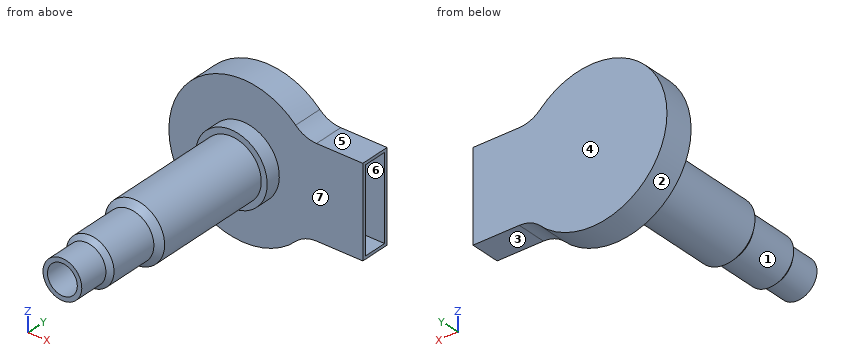
```python
from build123d import *

# Parameters (mm, degrees)
BOSS_EXTRUDE1_DEPTH = 10
SHELL1_T            = -1


with BuildPart() as part:
    # Sketch1 → Revolve1 (revolve)
    with BuildSketch(Plane(origin=(0, 0, 0), x_dir=(0, 0, -1), z_dir=(1, 0, 0))):
        Polygon((5, 0), (6.5, 0), (6.5, 10), (8, 11.5), (8, 28), (10, 30), (10, 70), (12, 70), (12, 75), (0, 75), (0, 35), (5, 35), align=None)
    revolve(axis=Axis((0, 0, 0), (0, 1, 0)))


with BuildPart() as body_2:
    # Sketch2 → Boss-Extrude1 (new body)
    with BuildSketch(Plane(origin=(0, 75, 0), x_dir=(1, 0, 0), z_dir=(0, 1, 0))):
        with BuildLine():
            Line((24.494897428, 15), (40, 15))
            Line((40, 15), (40, -15))
            Line((40, -15), (24.494897428, -15))
            ThreePointArc((24.494897428, -15), (20.715252698, -15.741799002), (17.496355306, -17.857142857))
            ThreePointArc((17.496355306, -17.857142857), (-25, 0), (17.496355306, 17.857142857))
            ThreePointArc((17.496355306, 17.857142857), (20.715252698, 15.741799002), (24.494897428, 15))
        make_face()
    extrude(amount=BOSS_EXTRUDE1_DEPTH)

    # Shell1
    shell1_openings = [body_2.faces().sort_by_distance(p)[0] for p in [
        (40, 80, 0),
    ]]
    offset(amount=SHELL1_T, openings=shell1_openings, kind=Kind.INTERSECTION)

    # Combine1: union part
    add(part.part)


solid = body_2.part
```
Source: CAD feature listing. Evaluate the final solid. Frame: model axes, mm. Face numbers are marked on the shaded views. A direction names the side the tool comes from. Round coordinates to 2 decimals unless told otherwise and drop trailing zeros. Loops run counter-clockwise (first coordinate to the right, second up) from the corner with the lowest first, then second, coordinate; pieces in that order, holes last.
(1) Section query C-C (z = -19.5). Output: boundary loops of the cut face in (x, y).
From the geometry:
outline: (-15.64, 75) - (15.64, 75) - (15.64, 85) - (-15.64, 85) - close; hole (-13.99, 76) - (13.99, 76) - (13.99, 84) - (-13.99, 84) - close
(2) Section query B-B (z = 0). Output: boundary loops of the cut face in (x, y), and give its area (3 significant figures).
From the geometry:
outline: (-25, 75) - (-12, 75) - (-12, 70) - (-10, 70) - (-10, 30) - (-8, 28) - (-8, 11.5) - (-6.5, 10) - (-6.5, 0) - (-5, 0) - (-5, 35) - (5, 35) - (5, 0) - (6.5, 0) - (6.5, 10) - (8, 11.5) - (8, 28) - (10, 30) - (10, 70) - (12, 70) - (12, 75) - (40, 75) - (40, 76) - (-24, 76) - (-24, 84) - (40, 84) - (40, 85) - (-25, 85) - close
area: 1,160 mm2
(3) Section query D-D (y = 13). Output: boundary loops of the cut face in (x, z).
From the geometry:
outline: circle Ø16 at (0, 0); hole circle Ø10 at (0, 0)
(4) Contact query for flat-ended pins moving along their axis: pin 1 Ø4 at (y, z) = (72, 10) entering from +X; pin 2 Ø9 at (x, y) = (34.5, 81.5) entering from +Z; pin 3 Ø5 at (x, y) = (30, 82.5) entering from -Z. Output: stop coordinate, or through.
From the geometry:
pin 1: stops at x = 8.94
pin 2: stops at z = 15
pin 3: stops at z = -15
(5) Access query for the marked faces 1, 2 and 3. Directions: +Z, -Z, +X, -X, +Y, -Y. A direction counts if a zero-diameter tool reaches every point of the face in a straight line with its end or side. Return the directions, or none.
From the geometry:
face 1: -Y
face 2: +Y, -Y
face 3: -Z, +X, +Y, -Y
(6) Pull-direction query (Y, two-part tool) for the marked faces 4, 5, 6 and 7; classes: +Y half, -Y half, draft (parallel to the pull), parting line (faces both ways), or undercut.
From the geometry:
face 4: +Y half
face 5: draft
face 6: undercut
face 7: -Y half
(7) Section query A-A (x = 0). Output: boundary loops of the cut face in (y, z), and give its area (3 significant figures).
From the geometry:
outline: (0, -6.5) - (10, -6.5) - (11.5, -8) - (28, -8) - (30, -10) - (70, -10) - (70, -12) - (75, -12) - (75, -25) - (85, -25) - (85, 25) - (75, 25) - (75, 12) - (70, 12) - (70, 10) - (30, 10) - (28, 8) - (11.5, 8) - (10, 6.5) - (0, 6.5) - (0, 5) - (35, 5) - (35, -5) - (0, -5) - close; hole (76, -24) - (84, -24) - (84, 24) - (76, 24) - close
area: 1,140 mm2
(8) Material intervals for probe 1 along Y at (x, z) = (10.5, 0); probe 2 along Z at (x, y) = (0, 18.5); probe 3 along Y at (x, z) = (14.5, -7.5), sorted ascending.
From the geometry:
probe 1: y = 70 to 76, 84 to 85
probe 2: z = -8 to -5, 5 to 8
probe 3: y = 75 to 76, 84 to 85
